```python
from build123d import *

# Parameters (mm, degrees)
BOSS_EXTRUDE1_DEPTH = 5.08
SKETCH2_R           = 1.905
CUT_EXTRUDE1_DEPTH  = 6.08
SKETCH5_W           = 15.24
SKETCH5_H           = 5.08
CUT_EXTRUDE2_DEPTH  = 21.32


with BuildPart() as part:
    # Sketch1 → Boss-Extrude1 (new body)
    with BuildSketch(Plane.XY):
        Polygon((0, 0), (63.5, 0), (31.75, 25.4), align=None)
    extrude(amount=BOSS_EXTRUDE1_DEPTH)

    # Sketch2 → Cut-Extrude1 (cut, through all)
    with BuildSketch(Plane.XY.offset(5.08)):
        with Locations((14.481967782, 5.08)):
            Circle(SKETCH2_R)
        with Locations((49.018032218, 5.08)):
            Circle(SKETCH2_R)
    extrude(amount=-CUT_EXTRUDE1_DEPTH, mode=Mode.SUBTRACT)

    # Sketch5 → Cut-Extrude2 (cut, through all)
    with BuildSketch(Plane(origin=(0, 5.08, 0), x_dir=(-1, 0, 0), z_dir=(0, -1, 0))):
        with Locations((-31.75, -2.54)):
            Rectangle(SKETCH5_W, SKETCH5_H)
    extrude(amount=-CUT_EXTRUDE2_DEPTH, mode=Mode.SUBTRACT)


solid = part.part
```
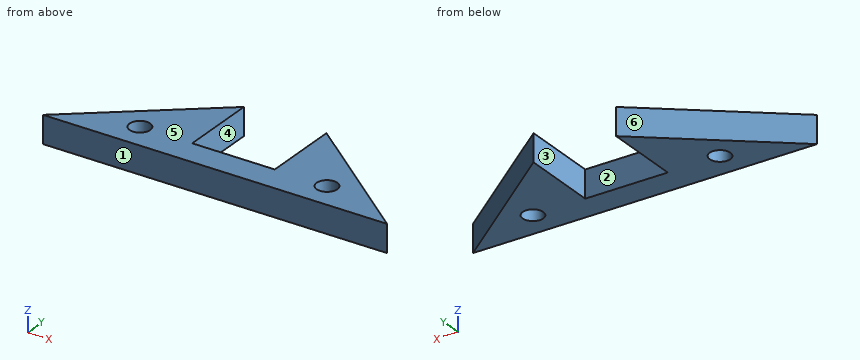
Design review of the part built by this model. Coordinates are the model's own, in mm. Face numbers are marked on the shaded views. A direction names the side the tool comes from. Round coordinates to 2 decimals unless told otherwise and drop trailing zeros. Order: outer loops, then holes, each group sorted by start corner. A loop starts at its lowest first (then second) coordinate and runs counter-clockwise, first axis right, second up. Notation, with made-up numbers: M 5.5,-17 L 43.5,-17 A12 ccw 43.5,2 Z; hole C 47,33 d8. An arc over 180 degrees is marked long. Put each result on its own line as item: value.
Q1. Draft analysis for pull direction X (two halves, no side actions). For the marked faces 3, 4, 5 and 6, state which applies: released by +X, released by -X, zero draft, split by the parting line, or undercut.
Reported:
face 3: undercut
face 4: undercut
face 5: zero draft
face 6: released by -X
Q2. Consider section A-A (z = 1.9). State the section outline as (x, y) points (3 decimals).
Reported:
outline: M 0,0 L 63.5,0 L 39.37,19.304 L 39.37,5.08 L 24.13,5.08 L 24.13,19.304 Z; hole C 14.482,5.08 d3.81; hole C 49.018,5.08 d3.81
Q3. Insertion check: pin 1 Ø2.5 at (x, z) = (28.5, 2.5) entering from +Y. The pin has a flat end and moves straight along its axis. Give the tip position at first contact, or say it passes through.
Reported:
pin 1: y = 5.08
Q4. To check wall thickness, follow line 1 (X direction, y = 4.25, z = 0.4); line 2 (X direction, y = 6.5, z = 2.1) (3 decimals); line 3 (X direction, y = 6, z = 3.6). State the ranges of each line that lie inside material, in increasing order.
Reported:
line 1: 5.31 to 12.77, 16.2 to 47.3, 50.73 to 58.19
line 2: 8.125 to 13.212, 15.752 to 24.13, 39.37 to 47.748, 50.288 to 55.375
line 3: 7.5 to 12.81, 16.15 to 24.13, 39.37 to 47.35, 50.69 to 56
Q5. Machinability: for the marked faces 1 and 2, which of the approach directions +Z, -Z, +X, -X, +Y, -Y give a long, thin tool a straight path to every point of the face, cutting with its end or side? Answer none if there is none.
Reported:
face 1: +Z, -Z, +X, -X, -Y
face 2: +Z, -Z, +Y
Q6. Consider section D-D (x = 8.5). State the section outline as (y, z) points.
Reported:
outline: M 0,0 L 6.8,0 L 6.8,5.08 L 0,5.08 Z
Q7. Consider section C-C (y = 4.5). State the section outline as (x, z) points (3 decimals).
Reported:
outline: M 5.625,0 L 12.667,0 L 12.667,5.08 L 5.625,5.08 Z; M 16.297,0 L 47.203,0 L 47.203,5.08 L 16.297,5.08 Z; M 50.833,0 L 57.875,0 L 57.875,5.08 L 50.833,5.08 Z
Q8. Consider section B-B (y = 15). State the section outline as (x, z) points.
Reported:
outline: M 18.75,0 L 24.13,0 L 24.13,5.08 L 18.75,5.08 Z; M 39.37,0 L 44.75,0 L 44.75,5.08 L 39.37,5.08 Z
